from build123d import *

# Parameters (mm, degrees)
SKETCH_1_R          = 10.9
EXTRUDE_1_DEPTH     = 1
DOME_1_FACE_RADIUS  = 10.9
DOME_1_HEIGHT       = 2.5
SKETCH_2_R          = 9.5
EXTRUDE_2_DEPTH     = 12.5
SKETCH_3_R          = 8.85
EXTRUDE_3_DEPTH     = 15.4
SKETCH_4_R          = 7.35
EXTRUDE_4_DEPTH     = 17.5
EXTRUDE_START       = -17.5
SKETCH_6_W          = 5
SKETCH_6_H          = 5
EXTRUDE_5_DEPTH     = 6
EXTRUDE_5_DRAFT     = -1
SKETCH_7_W          = 4
SKETCH_7_H          = 4
EXTRUDE_6_DEPTH     = 4.5
EXTRUDE_START_2     = -22
SKETCH_8_R          = 1.5
EXTRUDE_7_DEPTH     = 1
EXTRUDE_START_3     = -23
SKETCH_9_R          = 2
EXTRUDE_11_DEPTH    = 1.6
CUT_EXTRUDE_START   = 5
SKETCH_5_R          = 7.1
SKETCH_5_R_2        = 7
CUT_EXTRUDE_1_DEPTH = 15


with BuildPart() as part:
    # Эскиз1 → Бобышка-Вытянуть1 (new body)
    with BuildSketch(Plane(origin=(0, 0, 0), x_dir=(1, 0, 0), z_dir=(0, 1, 0))):
        with Locations(Location((0, 0, 0), (0, 0, 270))):
            Circle(SKETCH_1_R)
    extrude(amount=EXTRUDE_1_DEPTH)

    # Купол1: a dome of height H over a round flat face of radius A is a cap of a sphere of radius (A * A + H * H) / (2 * H)
    dome_1_r = (DOME_1_FACE_RADIUS * DOME_1_FACE_RADIUS + DOME_1_HEIGHT * DOME_1_HEIGHT) / (2 * DOME_1_HEIGHT)
    dome_1_base = Plane((0, 1, 0), z_dir=(0, 1, 0))
    with Locations(dome_1_base.offset(DOME_1_HEIGHT - dome_1_r)):
        dome_1_ball = Sphere(dome_1_r, mode=Mode.PRIVATE)
    add(split(dome_1_ball, bisect_by=dome_1_base, keep=Keep.TOP, mode=Mode.PRIVATE))

    # Эскиз2 → Бобышка-Вытянуть2 (add)
    with BuildSketch(Plane(origin=(0, 0, 0), x_dir=(1, 0, 0), z_dir=(0, 1, 0))):
        with Locations(Location((0, 0, 0), (0, 0, 270))):
            Circle(SKETCH_2_R)
    extrude(amount=-EXTRUDE_2_DEPTH)

    # Эскиз3 → Бобышка-Вытянуть3 (add)
    with BuildSketch(Plane(origin=(0, 0, 0), x_dir=(1, 0, 0), z_dir=(0, 1, 0))):
        with Locations(Location((0, 0, 0), (0, 0, 270))):
            Circle(SKETCH_3_R)
    extrude(amount=-EXTRUDE_3_DEPTH)

    # Эскиз4 → Бобышка-Вытянуть4 (add)
    with BuildSketch(Plane(origin=(0, 0, 0), x_dir=(1, 0, 0), z_dir=(0, 1, 0))):
        with Locations(Location((0, 0, 0), (0, 0, 270))):
            Circle(SKETCH_4_R)
    extrude(amount=-EXTRUDE_4_DEPTH)


with BuildPart() as extrude_5_tool:
    # Эскиз6 → Бобышка-Вытянуть5 (with draft: the straight prism first)
    with BuildSketch(Plane(origin=(0, 0, 0), x_dir=(1, 0, 0), z_dir=(0, 1, 0)).offset(EXTRUDE_START)):
        Rectangle(SKETCH_6_W, SKETCH_6_H)
    extrude(amount=-EXTRUDE_5_DEPTH)
    # Бобышка-Вытянуть5: the draft: its side faces are tilted about the plane it starts from
    extrude_5_sides = [extrude_5_tool.faces().sort_by_distance(p)[0] for p in [
        (0, -20.5, 2.5),
        (2.5, -20.5, 0),
        (0, -20.5, -2.5),
        (-2.5, -20.5, 0),
    ]]
    draft(extrude_5_sides, Plane(origin=(0, 0, 0), x_dir=(1, 0, 0), z_dir=(0, 1, 0)).offset(EXTRUDE_START), EXTRUDE_5_DRAFT)


with BuildPart() as part_1:
    add(part.part)

    # Бобышка-Вытянуть5: add extrude_5_tool
    add(extrude_5_tool.part)

    # Эскиз7 → Бобышка-Вытянуть6 (add)
    with BuildSketch(Plane(origin=(0, 0, 0), x_dir=(1, 0, 0), z_dir=(0, 1, 0)).offset(EXTRUDE_START)):
        with Locations((-4.5, 0)):
            Rectangle(SKETCH_7_W, SKETCH_7_H)
    extrude_6 = extrude(amount=-EXTRUDE_6_DEPTH)

    # Зеркальное отражение1: Бобышка-Вытянуть6 across plane
    add(extrude_6.mirror(Plane(origin=(0, 0, 0), x_dir=(0, 0, 1), z_dir=(1, 0, 0))))

    # Эскиз8 → Бобышка-Вытянуть7 (add)
    with BuildSketch(Plane(origin=(0, 0, 0), x_dir=(1, 0, 0), z_dir=(0, 1, 0)).offset(EXTRUDE_START_2)):
        with Locations(Location((-4.5, 0, 0), (0, 0, 270))):
            Circle(SKETCH_8_R)
    extrude_7 = extrude(amount=-EXTRUDE_7_DEPTH)

    # Эскиз9 → Бобышка-Вытянуть11 (add)
    with BuildSketch(Plane(origin=(0, 0, 0), x_dir=(1, 0, 0), z_dir=(0, 1, 0)).offset(EXTRUDE_START_3)):
        with Locations(Location((-4.5, 0, 0), (0, 0, 270))):
            Circle(SKETCH_9_R)
    extrude_11 = extrude(amount=-EXTRUDE_11_DEPTH)

    # Зеркальное отражение3: Бобышка-Вытянуть7, Бобышка-Вытянуть11 across plane
    add(extrude_7.mirror(Plane(origin=(0, 0, 0), x_dir=(0, 0, 1), z_dir=(1, 0, 0))))
    add(extrude_11.mirror(Plane(origin=(0, 0, 0), x_dir=(0, 0, 1), z_dir=(1, 0, 0))))

    # Эскиз5 → Вырез-Вытянуть1 (cut)
    with BuildSketch(Plane(origin=(0, 0, 0), x_dir=(1, 0, 0), z_dir=(0, 1, 0)).offset(CUT_EXTRUDE_START)):
        with Locations(Location((0, 0, 0), (0, 0, 270))):
            Circle(SKETCH_5_R)
        with Locations(Location((0, 0, 0), (0, 0, 270))):
            Circle(SKETCH_5_R_2, mode=Mode.SUBTRACT)
    extrude(amount=-CUT_EXTRUDE_1_DEPTH, mode=Mode.SUBTRACT)


solid = part_1.part
Can you work these out from the model? Positions are in its coordinate system, mm. A direction names the side the tool comes from. Round coordinates to 2 decimals unless told otherwise and drop trailing zeros. Order: outer loops, then holes, each group sorted by start corner. A loop starts at its lowest first (then second) coordinate and runs counter-clockwise, first axis right, second up. Notation, with made-up numbers: M 46.25,48 L 54.25,48 A15 ccw 54.25,76 Z; hole C 79.25,45 d9. An arc over 180 degrees is marked long. Use a Markdown table: item, result.
1) Imagine slicing it at C-C (z = -8.25). List the corners of the cut face in (x, y) for me.
Geometry says:
| item | result |
|---|---|
| outline | M -7.12,0 L -4.71,0 L -4.71,-12.5 L -3.2,-12.5 L -3.2,-15.4 L 3.2,-15.4 L 3.2,-12.5 L 4.71,-12.5 L 4.71,0 L 7.12,0 L 7.12,1 A23.61 ccw -7.12,1 Z |
2) If we mould it in two halves opening along Y, with no side actions, what happens to faces 1 (the face through (3.013, -22.493, -0.195)), 2 (the face through (0, -23.5, 0)), 3 (the face through (-5.78, -6.16, -7.54))? For each: +Y half, -Y half, draft (parallel to the pull), parting line (faces both ways), or undercut.
Geometry says:
| item | result |
|---|---|
| face 1 | undercut |
| face 2 | -Y half |
| face 3 | draft |
3) Imagine slicing it at D-D (y = 1.5). List the corners of the cut face in (x, z) for me, then the cut area to 3 significant figures.
Geometry says:
| item | result |
|---|---|
| outline | C 0,0 d19.6; C 0,0 d14; hole C 0,0 d14.2 |
| area | 297 mm² |
4) If I drill on line 1 along Y through (x, z) = (0, 0.5) (3 decimals); line 2 along Z through (x, y) = (5.75, -18.5); line 3 along Z through (x, y) = (3, -23.25), over which ranges is the centre line in solid material (lowest first)?
Geometry says:
| item | result |
|---|---|
| line 1 | y = -23.5 to 3.495 |
| line 2 | z = -2 to 2 |
| line 3 | z = -1.32 to 1.32 |
5) I'm going to push flat-ended pins straight in: P1, Ø2, axis at x = 6, y = -2, coming from the +Z side; P2, Ø2, axis at x = -5.5, y = -19.5, coming from the -Z side; P3, Ø3, axis at x = 4, z = -0.5, coming from the +Y side. Where does each tip first touch, or does it pass through?
Geometry says:
| item | result |
|---|---|
| P1 | stops at z = 8.08 |
| P2 | stops at z = -2 |
| P3 | stops at y = 3.37 |
6) On a 3-axis mill with a long thin cutter (end or side, diameter ignored), from which of +Z, -Z, +X, -X, +Y, -Y can I reach the whole of each face in a straight line? I mean faces 4 (the face through (6.5, -20, 0)), 5 (the face through (-5, -20, -2)), 6 (the face through (-7.175, -16.435, -1.593)), 7 (the face through (3, -23, 1)), 8 (the face through (5, -20, -2)). Say none if no direction works.
Geometry says:
| item | result |
|---|---|
| face 4 | +Z, -Z, +X, -Y |
| face 5 | -Z, -X, -Y |
| face 6 | -Y |
| face 7 | none |
| face 8 | -Z, +X, -Y |
7) Imagine slicing it at B-B (x = 0). List the corners of the cut face in (y, z) for me.
Geometry says:
| item | result |
|---|---|
| outline | M -23.5,-2.4 L -17.5,-2.5 L -17.5,-7.35 L -15.4,-7.35 L -15.4,-8.85 L -12.5,-8.85 L -12.5,-9.5 L 0,-9.5 L 0,-10.9 L 1,-10.9 A25.01 ccw 2.47,-7.1 L -10,-7.1 L -10,-7 L 2.5,-7 A25.01 ccw 2.5,7 L -10,7 L -10,7.1 L 2.47,7.1 A25.01 ccw 1,10.9 L 0,10.9 L 0,9.5 L -12.5,9.5 L -12.5,8.85 L -15.4,8.85 L -15.4,7.35 L -17.5,7.35 L -17.5,2.5 L -23.5,2.4 Z |
8) Imagine slicing it at A-A (y = -21.5). List the corners of the cut face in (x, z) for me.
Geometry says:
| item | result |
|---|---|
| outline | M -6.5,-2 L -2.5,-2 L -2.5,2 L -6.5,2 Z; M -2.43,-2.43 L 2.43,-2.43 L 2.43,2.43 L -2.43,2.43 Z; M 2.5,-2 L 6.5,-2 L 6.5,2 L 2.5,2 Z |
